Drawing for the job (mm, zero at the part's lowest x, y, z). A direction names the side the tool comes from. Coordinates: 2 decimals unless noted, no trailing zeros. Write each loop counter-clockwise with the first axis right and the second up, starting at its lowest first coordinate (ties: lowest second). Pieces come first, ordered by that corner, then holes. Notation, with made-up numbers: M 42,75 L 68,75 A13 ccw 68,88 Z; hole C -4.75,-33.5 d2. An arc over 180 degrees is marked long. Put each result on its own line as item: value. Start each with the question number.
Q1. Drill centre lines: line 1 along Z through (x, y) = (9, 1.7); line 2 along Z through (x, y) = (19.5, 6); line 3 along Y through (x, z) = (6.25, 17). Where is each one in solid material? Low to high.
Q2. Pull direction Y, two halves, no side cores. Call the marked faces 1, 2 and 3: pulls with the +Y half, pulls with the -Y half, needs draft (parallel to the pull), parting line crosses it, or undercut.
Q3. Which spindle directions (+Z, -Z, +X, -X, +Y, -Y) get a long thin tool onto all of the face, cutting with end or side? Do the marked faces 4 and 5. Say none if no direction does.
Q4. Cut at D-D (x = 9). Write the cut outline in (y, z), then the cut area to 3 significant figures.
Q5. Cut at A-A (y = 26). Write the cut outline in (x, z), then the cut area to 3 significant figures.
Q6. Cut at C-C (z = 3.5). Write the cut outline in (x, y), then the cut area to 3 significant figures.
Q7. Drop a flat-ended pin along its axis: pin 1 (3.5 mm diameter, centred on y = 6, z = 3.5, fed in from -X). Give the stop position or say it passes through.
Q8. Cut at B-B (x = 17.25). Write the cut outline in (y, z), then the cut area to 3 significant figures.
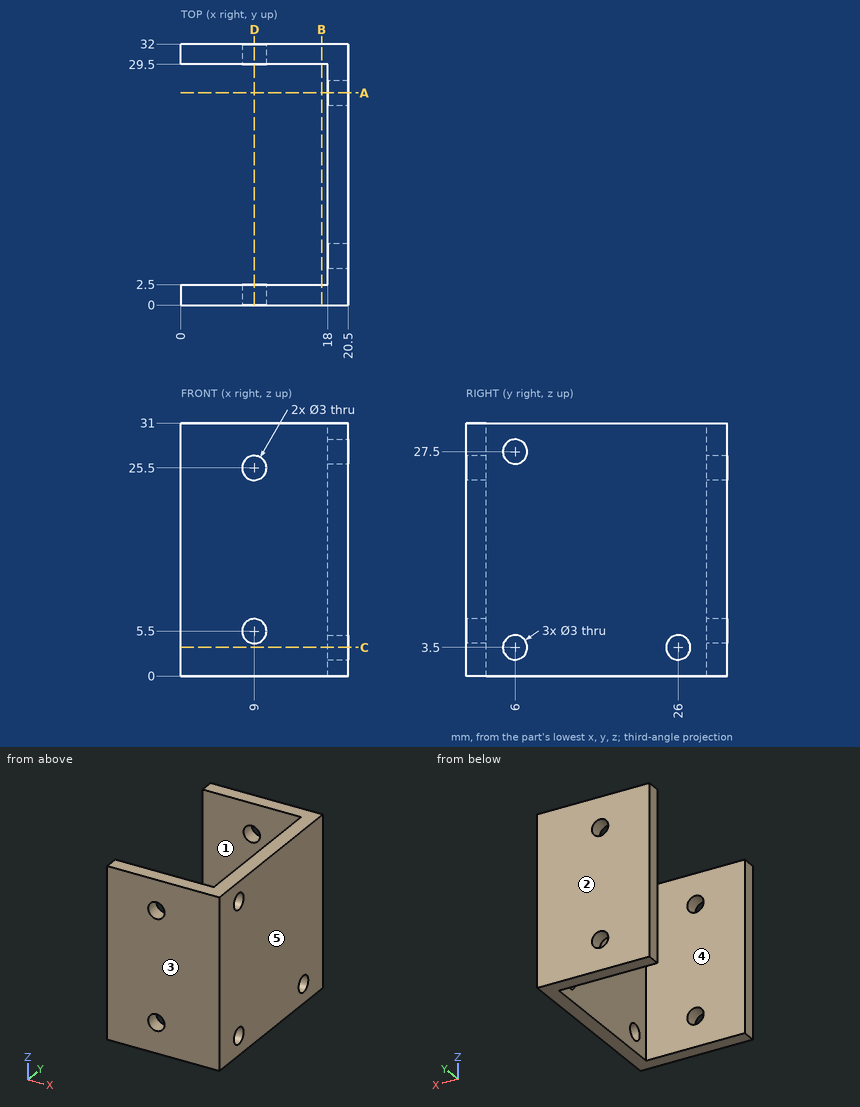
Computed values:
1. line 1: 0 to 4, 7 to 24, 27 to 31
1. line 2: 0 to 2, 5 to 26, 29 to 31
1. line 3: 0 to 2.5, 29.5 to 32
2. face 1: undercut
2. face 2: pulls with the +Y half
2. face 3: pulls with the -Y half
3. face 4: +Z, -Z, -X
3. face 5: +Z, -Z, +X, +Y, -Y
4. outline: M 0,0 L 2.5,0 L 2.5,4 L 0,4 Z; M 0,7 L 2.5,7 L 2.5,24 L 0,24 Z; M 0,27 L 2.5,27 L 2.5,31 L 0,31 Z; M 29.5,0 L 32,0 L 32,4 L 29.5,4 Z; M 29.5,7 L 32,7 L 32,24 L 29.5,24 Z; M 29.5,27 L 32,27 L 32,31 L 29.5,31 Z
4. area: 125 mm2
5. outline: M 18,0 L 20.5,0 L 20.5,2 L 18,2 Z; M 18,5 L 20.5,5 L 20.5,31 L 18,31 Z
5. area: 70.0 mm2
6. outline: M 0,0 L 20.5,0 L 20.5,4.5 L 18,4.5 L 18,2.5 L 0,2.5 Z; M 0,29.5 L 18,29.5 L 18,27.5 L 20.5,27.5 L 20.5,32 L 0,32 Z; M 18,7.5 L 20.5,7.5 L 20.5,24.5 L 18,24.5 Z
6. area: 155 mm2
7. pin 1: x = 18
8. outline: M 0,0 L 2.5,0 L 2.5,31 L 0,31 Z; M 29.5,0 L 32,0 L 32,31 L 29.5,31 Z
8. area: 155 mm2
